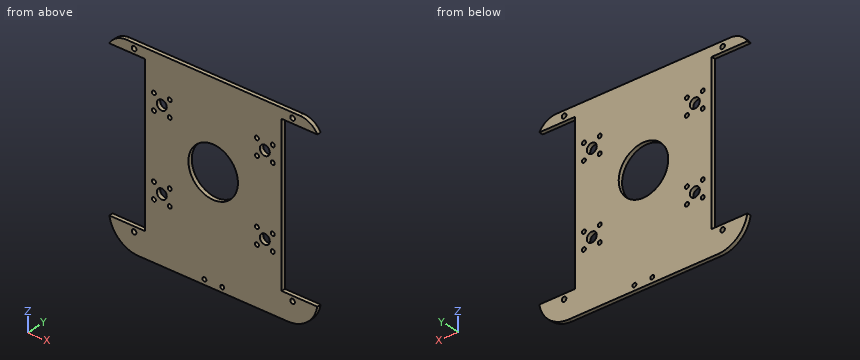
```python
from build123d import *

# Parameters (mm, degrees)
SKETCH1_R           = 25
SKETCH1_R_2         = 2
SKETCH1_R_3         = 2.32
SKETCH1_R_4         = 5
BOSS_EXTRUDE1_DEPTH = 4
FILLET1_R           = 30
FILLET2_R           = 20


with BuildPart() as part:
    # Sketch1 → Boss-Extrude1 (new body)
    with BuildSketch(Plane(origin=(0, 0, 0), x_dir=(1, 0, 0), z_dir=(0, 1, 0))):
        Polygon((-153.14810061, 80), (-117.14810061, 80), (-117.14810061, -75), (-153.14810061, -75), (-153.14810061, -85), (56.85189939, -85), (56.85189939, -75), (20.85189939, -75), (20.85189939, 80), (56.85189939, 80), (56.85189939, 105), (-153.14810061, 105), align=None)
        with Locations(Location((-48.295998841, 0.000104161, 0), (0, 0, 270))):
            Circle(SKETCH1_R, mode=Mode.SUBTRACT)
        with Locations(Location((-57.14810061, 100, 0), (0, 0, 270))):
            Circle(SKETCH1_R_2, mode=Mode.SUBTRACT)
        with Locations(Location((-39.14810061, 100, 0), (0, 0, 90))):
            Circle(SKETCH1_R_2, mode=Mode.SUBTRACT)
        with Locations(Location((-128.14810061, -80, 0), (0, 0, 270))):
            Circle(SKETCH1_R_3, mode=Mode.SUBTRACT)
        with Locations(Location((-128.14810061, 85, 0), (0, 0, 90))):
            Circle(SKETCH1_R_3, mode=Mode.SUBTRACT)
        with Locations(Location((31.85189939, 85, 0), (0, 0, 270))):
            Circle(SKETCH1_R_3, mode=Mode.SUBTRACT)
        with Locations(Location((31.85189939, -80, 0), (0, 0, 90))):
            Circle(SKETCH1_R_3, mode=Mode.SUBTRACT)
        with Locations(Location((-108.14810061, -48, 0), (0, 0, 270))):
            Circle(SKETCH1_R_2, mode=Mode.SUBTRACT)
        with Locations(Location((-92.14810061, -48, 0), (0, 0, 270))):
            Circle(SKETCH1_R_2, mode=Mode.SUBTRACT)
        with Locations(Location((-92.14810061, -32, 0), (0, 0, 90))):
            Circle(SKETCH1_R_2, mode=Mode.SUBTRACT)
        with Locations(Location((-108.14810061, -32, 0), (0, 0, 90))):
            Circle(SKETCH1_R_2, mode=Mode.SUBTRACT)
        with Locations(Location((-100.14810061, -40, 0), (0, 0, 270))):
            Circle(SKETCH1_R_4, mode=Mode.SUBTRACT)
        with Locations(Location((-92.14810061, 48, 0), (0, 0, 90))):
            Circle(SKETCH1_R_2, mode=Mode.SUBTRACT)
        with Locations(Location((-108.14810061, 48, 0), (0, 0, 90))):
            Circle(SKETCH1_R_2, mode=Mode.SUBTRACT)
        with Locations(Location((-92.14810061, 32, 0), (0, 0, 270))):
            Circle(SKETCH1_R_2, mode=Mode.SUBTRACT)
        with Locations(Location((-100.14810061, 40, 0), (0, 0, 90))):
            Circle(SKETCH1_R_4, mode=Mode.SUBTRACT)
        with Locations(Location((-108.14810061, 32, 0), (0, 0, 270))):
            Circle(SKETCH1_R_2, mode=Mode.SUBTRACT)
        with Locations(Location((-4.14810061, -32, 0), (0, 0, 270))):
            Circle(SKETCH1_R_2, mode=Mode.SUBTRACT)
        with Locations(Location((-4.14810061, -48, 0), (0, 0, 90))):
            Circle(SKETCH1_R_2, mode=Mode.SUBTRACT)
        with Locations(Location((3.85189939, -40, 0), (0, 0, 90))):
            Circle(SKETCH1_R_4, mode=Mode.SUBTRACT)
        with Locations(Location((11.85189939, -48, 0), (0, 0, 90))):
            Circle(SKETCH1_R_2, mode=Mode.SUBTRACT)
        with Locations(Location((11.85189939, -32, 0), (0, 0, 270))):
            Circle(SKETCH1_R_2, mode=Mode.SUBTRACT)
        with Locations(Location((-4.14810061, 32, 0), (0, 0, 90))):
            Circle(SKETCH1_R_2, mode=Mode.SUBTRACT)
        with Locations(Location((-4.14810061, 48, 0), (0, 0, 270))):
            Circle(SKETCH1_R_2, mode=Mode.SUBTRACT)
        with Locations(Location((11.85189939, 32, 0), (0, 0, 90))):
            Circle(SKETCH1_R_2, mode=Mode.SUBTRACT)
        with Locations(Location((11.85189939, 48, 0), (0, 0, 270))):
            Circle(SKETCH1_R_2, mode=Mode.SUBTRACT)
        with Locations(Location((3.85189939, 40, 0), (0, 0, 270))):
            Circle(SKETCH1_R_4, mode=Mode.SUBTRACT)
    extrude(amount=BOSS_EXTRUDE1_DEPTH)

    # Fillet1
    # the kernel refuses this fillet: 30 mm, written as the material it takes off along each edge
    with BuildSketch(Plane(origin=(56.85189939, -73.950997289, -105), x_dir=(0, 0, 1), z_dir=(0, 1, 0))) as fillet1_piece_1:
        with BuildLine():
            CenterArc((30, -29.580398915), FILLET1_R, 99.594068227, 80.405931773)
            Line((0, -29.580398916), (-0.6, -29.580398916))
            Line((-0.6, -29.580398916), (-0.6, 0))
            Line((-0.6, 0), (0, 0.6))
            ThreePointArc((0, 0.6), (12.5, 0.6), (24.9, 0.591607978))
            Line((24.9, 0.591607978), (25, 0))
        make_face()
    extrude(amount=151.901994578, mode=Mode.SUBTRACT)
    with BuildSketch(Plane(origin=(-153.14810061, -73.950997289, -105), x_dir=(1, 0, 0), z_dir=(0, 1, 0))) as fillet1_piece_2:
        with BuildLine():
            CenterArc((29.580398916, -30), FILLET1_R, 90, 80.405931773)
            Line((0, -25), (-0.591607978, -24.9))
            ThreePointArc((-0.591607978, -24.9), (-0.6, -12.5), (-0.6, 0))
            Line((-0.6, 0), (0, 0.6))
            Line((0, 0.6), (29.580398916, 0.6))
            Line((29.580398916, 0.6), (29.580398916, 0))
        make_face()
    extrude(amount=151.901994578, mode=Mode.SUBTRACT)

    # Fillet2
    # the kernel refuses this fillet: 20 mm, written as the material it takes off along each edge
    with BuildSketch(Plane(origin=(56.85189939, -43.301270189, 85), x_dir=(0, 0, -1), z_dir=(0, 1, 0))) as fillet2_piece_1:
        with BuildLine():
            CenterArc((20, 17.320508076), FILLET2_R, 180, 60)
            Line((0, 17.320508076), (-0.4, 17.320508076))
            Line((-0.4, 17.320508076), (-0.4, 0))
            Line((-0.4, 0), (0, -0.4))
            ThreePointArc((0, -0.4), (5, -0.4), (9.8, -0.346410162))
            Line((9.8, -0.346410162), (10, 0))
        make_face()
    extrude(amount=90.602540378, mode=Mode.SUBTRACT)
    with BuildSketch(Plane(origin=(-153.14810061, -43.301270189, 85), x_dir=(1, 0, 0), z_dir=(0, 1, 0))) as fillet2_piece_2:
        with BuildLine():
            CenterArc((17.320508076, 20), FILLET2_R, 210, 60)
            Line((0, 10), (-0.346410162, 9.8))
            ThreePointArc((-0.346410162, 9.8), (-0.4, 5), (-0.4, 0))
            Line((-0.4, 0), (0, -0.4))
            Line((0, -0.4), (17.320508076, -0.4))
            Line((17.320508076, -0.4), (17.320508076, 0))
        make_face()
    extrude(amount=90.602540378, mode=Mode.SUBTRACT)


solid = part.part
```
Source: CAD feature listing. Evaluate the final solid. Frame: model axes, mm. Coordinates: 2 decimals unless noted, no trailing zeros. Loops run counter-clockwise (first coordinate to the right, second up) from the corner with the lowest first, then second, coordinate; pieces in that order, holes last. Notation, with made-up numbers: (52, -3.5) -> (68, -3.5) arc R24 ccw to (68, 35.5) -> close; hole circle Ø2 at (23, 8.25). An arc over 180 degrees is marked (long way). One line per item, written item: value. Start each with the question number.
Q1. Contact query for flat-ended pins moving along their axis: P1, Ø8, axis at x = 3.85, z = -40, coming from the -Y side; P2, Ø2, axis at y = 1, z = 21.5, coming from the -X side. Output: stop coordinate, or through.
Q2. Section query A-A, the plane z = -40. Return the cut outline in (x, y), and give its area (3 significant figures).
Q3. Section query C-C, the plane z = -85. Return the cut outline in (x, y).
Q4. Section query B-B, the plane x = 25. Return the cut outline in (y, z), and give its area (3 significant figures).
Q5. Line query: line 1 along X through (y, z) = (1.6, -40); line 2 along X through (y, z) = (2.2, -32); line 3 along Z through (x, y) = (-129, 2.85). Output: solid intervals per line, ascending.
Q6. Section query D-D, the plane z = 68.5. Return the cut outline in (x, y), and give its area (3 significant figures).
Results:
1. P1: through
1. P2: x = -117.15
2. outline: (-117.15, 0) -> (-105.15, 0) -> (-105.15, 4) -> (-117.15, 4) -> close; (-95.15, 0) -> (-1.15, 0) -> (-1.15, 4) -> (-95.15, 4) -> close; (8.85, 0) -> (20.85, 0) -> (20.85, 4) -> (8.85, 4) -> close
2. area: 472 mm^2
3. outline: (-151.85, 0) -> (-130.47, 0) -> (-130.47, 4) -> (-151.85, 4) -> close; (-125.83, 0) -> (29.53, 0) -> (29.53, 4) -> (-125.83, 4) -> close; (34.17, 0) -> (55.56, 0) -> (55.56, 4) -> (34.17, 4) -> close
4. outline: (0, -105) -> (4, -105) -> (4, -80) -> (0, -80) -> close; (0, 75) -> (4, 75) -> (4, 85) -> (0, 85) -> close
4. area: 140 mm^2
5. line 1: -117.15 to -105.15, -95.15 to -1.15, 8.85 to 20.85
5. line 2: -117.15 to -110.15, -106.15 to -94.15, -90.15 to -6.15, -2.15 to 9.85, 13.85 to 20.85
5. line 3: -104.5 to -87.16, -82.84 to -80, 75 to 77.84, 82.16 to 85
6. outline: (-117.15, 0) -> (20.85, 0) -> (20.85, 4) -> (-117.15, 4) -> close
6. area: 552 mm^2
